Autodesk Inventor part; units mm, degrees
ref_plane "YZ Plane" through (0, 0, 0) normal (1, 0, 0) x (0, 1, 0)
ref_plane "XZ Plane" through (0, 0, 0) normal (0, 1, 0) x (-1, 0, 0)
ref_plane "XY Plane" through (0, 0, 0) normal (0, 0, 1) x (1, 0, 0)
sketch "スケッチ1" plane through (0, 0, 0) normal (0, 0, 1) x (1, 0, 0)
  circle A0 centre (55.7151, -22.426) radius 1
  circle A1 centre (55.7151, -6.426) radius 1.05
  circle A2 centre (20.7151, -6.426) radius 1
  circle A3 centre (4.7151, -6.426) radius 1.45
  circle A4 centre (-30.2849, -22.426) radius 1
  circle A5 centre (-30.2849, -6.426) radius 1.05
  circle A6 centre (55.7151, -22.426) radius 1.1
  circle A7 centre (55.7151, -6.426) radius 1.1
  circle A8 centre (20.7151, -6.426) radius 1.1
  circle A9 centre (4.7151, -6.426) radius 1.1
  circle A10 centre (-30.2849, -6.426) radius 1.1
  circle A11 centre (-30.2849, -22.426) radius 1.1
  circle A12 centre (20.7151, -42.426) radius 1
  circle A13 centre (4.7151, -42.426) radius 1
  circle A14 centre (20.7151, -42.426) radius 1.1
  circle A15 centre (4.7151, -42.426) radius 1.1
  circle A16 centre (55.7151, -6.426) radius 2.5
  circle A17 centre (-30.2849, -6.426) radius 2.5
  circle A18 centre (-30.2849, -22.426) radius 2.5
  circle A19 centre (55.7151, -22.426) radius 2.5
  circle A20 centre (20.7151, -42.426) radius 2.5
  circle A21 centre (4.7151, -42.426) radius 2.5
  line L0 (21.9554, -44.5966) -> (56.9554, -24.5966)
  line L1 (58.2151, -22.426) -> (58.2151, -6.426)
  line L2 (55.7151, -3.926) -> (-30.2849, -3.926)
  line L3 (-32.7849, -6.426) -> (-32.7849, -22.426)
  line L4 (3.4747, -44.5966) -> (-31.5253, -24.5966)
  line L5 (20.7151, -44.926) -> (4.7151, -44.926)
  circle A22 centre (91.7151, -22.426) radius 1
  circle A23 centre (91.7151, -22.426) radius 1.1
  circle A24 centre (-66.2849, -22.426) radius 1.05
  circle A25 centre (-66.2849, -22.426) radius 1.1
  circle A26 centre (-66.2849, -22.426) radius 2.5
  circle A27 centre (91.7151, -22.426) radius 2.5
  line L6 (92.3929, -24.8324) -> (21.3929, -44.8324)
  line L7 (91.7151, -19.926) -> (55.7151, -19.926)
  line L8 (73.8937, -20.8546) -> (67.5365, -20.8546)
  line L9 (73.8937, -16.9974) -> (73.8937, -20.8546)
  line L10 (67.5365, -16.9974) -> (73.8937, -16.9974)
  line L11 (67.5365, -20.8546) -> (67.5365, -16.9974)
  line L12 (73.8937, -20.8546) -> (67.5365, -20.8546)
  line L13 (67.6151, -17.226) -> (73.6151, -17.226)
  line L14 (73.6151, -17.226) -> (73.6151, -20.726)
  line L15 (73.6151, -20.726) -> (67.6151, -20.726)
  line L16 (67.6151, -20.726) -> (67.6151, -17.226)
  line L17 (65.6151, -22.726) -> (75.6151, -22.726)
  line L18 (75.6151, -22.726) -> (75.6151, -15.226)
  line L19 (75.6151, -15.226) -> (65.6151, -15.226)
  line L20 (65.6151, -15.226) -> (65.6151, -22.726)
  line L21 (-66.9603, -24.833) -> (3.4747, -44.5966)
  line L22 (-30.2849, -19.926) -> (-66.2849, -19.926)
  line L23 (-48.4635, -20.8546) -> (-48.4635, -16.9974)
  line L24 (-28.7849, -24.426) -> (-67.7849, -24.426)
  arc A28 (-28.7849, -24.426) -> (-28.2849, -23.926) centre (-28.7849, -23.926) ccw
  line L25 (-28.2849, -4.926) -> (-28.2849, -23.926)
  arc A29 (-28.2849, -4.926) -> (-28.7849, -4.426) centre (-28.7849, -4.926) ccw
  line L26 (-67.7849, -4.426) -> (-28.7849, -4.426)
  arc A30 (-67.7849, -4.426) -> (-68.2849, -4.926) centre (-67.7849, -4.926) ccw
  line L27 (-68.2849, -23.926) -> (-68.2849, -4.926)
  arc A31 (-68.2849, -23.926) -> (-67.7849, -24.426) centre (-67.7849, -23.926) ccw
  line L28 (-48.4635, -7.9974) -> (-42.1063, -7.9974)
  line L29 (-42.1063, -7.9974) -> (-42.1063, -11.8546)
  line L30 (-42.1063, -11.8546) -> (-48.4635, -11.8546)
  line L31 (-48.4635, -11.8546) -> (-48.4635, -7.9974)
  circle A32 centre (-40.8849, -14.426) radius 1.1519
  line L32 (-48.4635, -20.8546) -> (-48.4635, -16.9974)
  line L33 (-48.4635, -16.9974) -> (-42.1063, -16.9974)
  line L34 (-42.1063, -16.9974) -> (-42.1063, -20.8546)
  line L35 (-42.1063, -20.8546) -> (-48.4635, -20.8546)
  circle A33 centre (-66.2849, -6.426) radius 1.8131
  circle A34 centre (-66.2849, -22.426) radius 1.8131
  circle A35 centre (-30.2849, -6.426) radius 1.8131
  circle A36 centre (-30.2849, -22.426) radius 1.8131
  arc A37 (-59.7956, -8.176) -> (-59.7849, -20.676) centre (-59.7849, -14.426) ccw
  arc A38 (-60.0349, -7.926) -> (-59.7956, -8.1758) centre (-59.7849, -7.926) ccw
  line L36 (-60.0349, -7.926) -> (-60.0349, -6.176)
  arc A39 (-59.5349, -6.176) -> (-60.0349, -6.176) centre (-59.7849, -6.176) ccw
  line L37 (-59.5349, -6.176) -> (-59.5349, -7.926)
  arc A40 (-59.7849, -8.176) -> (-59.5349, -7.926) centre (-59.7849, -7.926) ccw
  arc A41 (-57.3931, -8.6518) -> (-59.7849, -8.176) centre (-59.7849, -14.426) ccw
  arc A42 (-57.5284, -8.3251) -> (-57.3931, -8.6518) centre (-57.2975, -8.4208) ccw
  line L38 (-57.5284, -8.3251) -> (-56.8587, -6.7083)
  arc A43 (-56.3968, -6.8997) -> (-56.8587, -6.7083) centre (-56.6278, -6.804) ccw
  line L39 (-56.3968, -6.8997) -> (-57.0665, -8.5165)
  arc A44 (-57.3931, -8.6518) -> (-57.0665, -8.5165) centre (-57.2975, -8.4208) ccw
  arc A45 (-55.3655, -10.0066) -> (-57.3931, -8.6518) centre (-59.7849, -14.426) ccw
  arc A46 (-55.3655, -9.653) -> (-55.3655, -10.0066) centre (-55.1887, -9.8298) ccw
  line L40 (-55.3655, -9.653) -> (-54.1281, -8.4156)
  arc A47 (-53.7745, -8.7692) -> (-54.1281, -8.4156) centre (-53.9513, -8.5924) ccw
  line L41 (-53.7745, -8.7692) -> (-55.0119, -10.0066)
  arc A48 (-55.3655, -10.0066) -> (-55.0119, -10.0066) centre (-55.1887, -9.8298) ccw
  arc A49 (-54.0107, -12.0342) -> (-55.3655, -10.0066) centre (-59.7849, -14.426) ccw
  arc A50 (-53.8754, -11.7076) -> (-54.0107, -12.0342) centre (-53.7797, -11.9386) ccw
  line L42 (-53.8754, -11.7076) -> (-52.2586, -11.0379)
  arc A51 (-52.0672, -11.4998) -> (-52.2586, -11.0379) centre (-52.1629, -11.2689) ccw
  line L43 (-52.0672, -11.4998) -> (-53.684, -12.1695)
  arc A52 (-54.0107, -12.0342) -> (-53.684, -12.1695) centre (-53.7797, -11.9386) ccw
  arc A53 (-53.5349, -14.426) -> (-54.0107, -12.0342) centre (-59.7849, -14.426) ccw
  arc A54 (-53.2849, -14.176) -> (-53.5349, -14.426) centre (-53.2849, -14.426) ccw
  line L44 (-53.2849, -14.176) -> (-51.5349, -14.176)
  arc A55 (-51.5349, -14.676) -> (-51.5349, -14.176) centre (-51.5349, -14.426) ccw
  line L45 (-51.5349, -14.676) -> (-53.2849, -14.676)
  arc A56 (-53.5349, -14.426) -> (-53.2849, -14.676) centre (-53.2849, -14.426) ccw
  arc A57 (-54.0107, -16.8178) -> (-53.5349, -14.426) centre (-59.7849, -14.426) ccw
  arc A58 (-53.684, -16.6825) -> (-54.0107, -16.8178) centre (-53.7797, -16.9134) ccw
  line L46 (-53.684, -16.6825) -> (-52.0672, -17.3522)
  arc A59 (-52.2586, -17.8141) -> (-52.0672, -17.3522) centre (-52.1629, -17.5831) ccw
  line L47 (-52.2586, -17.8141) -> (-53.8754, -17.1444)
  arc A60 (-54.0107, -16.8178) -> (-53.8754, -17.1444) centre (-53.7797, -16.9134) ccw
  arc A61 (-55.3655, -18.8454) -> (-54.0107, -16.8178) centre (-59.7849, -14.426) ccw
  arc A62 (-55.0119, -18.8454) -> (-55.3655, -18.8454) centre (-55.1887, -19.0222) ccw
  line L48 (-55.0119, -18.8454) -> (-53.7745, -20.0829)
  arc A63 (-54.1281, -20.4364) -> (-53.7745, -20.0829) centre (-53.9513, -20.2596) ccw
  line L49 (-54.1281, -20.4364) -> (-55.3655, -19.199)
  arc A64 (-55.3655, -18.8454) -> (-55.3655, -19.199) centre (-55.1887, -19.0222) ccw
  arc A65 (-57.3931, -20.2003) -> (-55.3655, -18.8454) centre (-59.7849, -14.426) ccw
  arc A66 (-57.0665, -20.3356) -> (-57.3931, -20.2003) centre (-57.2975, -20.4312) ccw
  line L50 (-57.0665, -20.3356) -> (-56.3968, -21.9523)
  arc A67 (-56.8587, -22.1437) -> (-56.3968, -21.9523) centre (-56.6278, -22.048) ccw
  line L51 (-56.8587, -22.1437) -> (-57.5284, -20.5269)
  arc A68 (-57.3931, -20.2003) -> (-57.5284, -20.5269) centre (-57.2975, -20.4312) ccw
  arc A69 (-59.7849, -20.676) -> (-57.3931, -20.2003) centre (-59.7849, -14.426) ccw
  arc A70 (-59.5349, -20.926) -> (-59.7849, -20.676) centre (-59.7849, -20.926) ccw
  line L52 (-59.5349, -20.926) -> (-59.5349, -22.676)
  arc A71 (-60.0349, -22.676) -> (-59.5349, -22.676) centre (-59.7849, -22.676) ccw
  line L53 (-60.0349, -22.676) -> (-60.0349, -20.926)
  arc A72 (-59.7849, -20.676) -> (-60.0349, -20.926) centre (-59.7849, -20.926) ccw
  line L54 (-50.4635, -22.8546) -> (-40.1063, -22.8546)
  line L55 (-40.1063, -22.8546) -> (-40.1063, -14.9974)
  line L56 (-40.1063, -14.9974) -> (-50.4635, -14.9974)
  line L57 (-50.4635, -22.8546) -> (-50.4635, -14.9974)
  circle A73 centre (-59.7849, -14.426) radius 8
  circle A74 centre (85.2151, -14.426) radius 8
  point P0 (0, 0)
  point P1 (-32.7849, -19.926)
  point P2 (-40.1063, -19.926)
  point P3 (-50.4635, -19.926)
  point P4 (-53.9314, -19.926)
  point P5 (-54.3076, -20.2569)
  point P6 (-56.494, -21.7178)
  point P7 (-56.9559, -21.9091)
  point P8 (-59.5349, -22.4221)
  point P9 (-60.0349, -22.4221)
  point P10 (-65.4578, -20.0668)
  point P11 (65.6151, -19.926)
  point P12 (58.2151, -19.926)
  point P13 (90.888, -20.0668)
  point P14 (79.4056, -19.926)
  point P15 (75.6151, -19.926)
  dimension "d0" = 2.2
  dimension "d1" = 2.2
  dimension "d2" = 2.2
  dimension "d3" = 2.2
  dimension "d4" = 2.2
  dimension "d5" = 2.2
  dimension "d6" = 2.2
  dimension "d7" = 2.2
  dimension "d8" = 5
  dimension "d9" = 5
  dimension "d10" = 5
  dimension "d11" = 5
  dimension "d12" = 5
  dimension "d13" = 5
  dimension "d18" = 2.2
  dimension "d19" = 2.2
  dimension "d20" = 5
  dimension "d21" = 5
  dimension "d22" = 2
  dimension "d23" = 2
  dimension "d24" = 2
extrude "押し出し1" add sketch "スケッチ1" along normal blind 1.5 contours A3 | A16 | L1 L7 A19 L0 A20 L5 A21 L4 A18 A28 L25 A17 A29 L2 A16 | L7 L20 L17 L18 A74 A27 L6 A20 L0 A19 L1 | L1 A19 L7 | A17 L26 | A19 | A29 A17 | A17 L25 L26 | A17 L25 | A17 L25 A18 L22 L3 | A20 | L22 A18 L3 | L3 A18 L24 A26 A73 L53 A71 L52 L51 A67 L50 L49 A63 L48 L22 L57 L54 L55 | L25 A18 L24 | A18 L25 | L27 A26 | A26 A73 L24 L27 | A27 A74 | A28 A18 | L24 A18 | A18 L4 L21 A26 L24 | A21 | A26 L24 | A34 | A35 | A36 picked at (89.8821, -21.5749)
sketch "スケッチ2" plane through (0, 0, 1.5) normal (0, 0, 1) x (1, 0, 0)
  circle A0 centre (12.7151, -12.926) radius 8
  point P0 (0, 0)
extrude "押し出し2" cut sketch "スケッチ2" against normal through all
fillet "フィレット1" radius 2 8 edges at (75.6151, -19.926, 0.75) (75.6151, -22.726, 0.75) (65.6151, -22.726, 0.75) (65.6151, -19.926, 0.75) (-50.4635, -19.926, 0.75) (-50.4635, -22.8546, 0.75) (-40.1063, -22.8546, 0.75) (-40.1063, -19.926, 0.75)
properties part number "jouhansin_sita"
Geometry: final body of the model. Coordinates: model frame, mm. Coordinates: 2 decimals unless noted, no trailing zeros. Order: outer loops, then holes, each group sorted by start corner. A loop starts at its lowest first (then second) coordinate and runs counter-clockwise, first axis right, second up.
(1) First-contact query: pin 1 (2.5 mm diameter, centred on x = -30.28, y = -22.43, fed in from +Z); pin 2 (2 mm diameter, centred on x = 4.72, y = -42.43, fed in from +Z); pin 3 (0.8 mm diameter, centred on y = -11.5, z = 0.5, fed in from +X). Flat tips, straight axial feed; report the tip coordinate or a pass-through.
(2) Section query A-A (x = 17). Return the cut outline in (y, z).
(3) Draft query along Y for faces 1 (the face through (57.39, -34.692, 0.74)), 2 (the face through (12, -24, 0)), 3 (the face through (17.016, -6.18, 0.76)), 4 (the face through (-68.685, -21.728, 0.74)). Return one class per face: pulls with the +Y half, pulls with the -Y half, needs draft (parallel to the pull), parting line crosses it, or undercut.
(4) Section query B-B (y = -18). Return the cut outline in (x, z), plus the area to 3 significant figures.
(5) Section query C-C (z = 0.65). State how many separate pieces and enclosed holes the cut face has, plus the area to 3 significant figures.
(6) Material intervals for probe 1 along Y at (x, z) = (-30, 1.1); probe 2 along Y at (x, z) = (5.5, 0.5); probe 3 along Y at (x, z) = (56, 0.5), sorted ascending.
(7) Section query D-D (x = -11). Return the cut outline in (y, z), plus the area to 3 significant figures.
Solution:
1. pin 1: stops at z = 1.5
1. pin 2: passes through
1. pin 3: stops at x = 58.22
2. outline: (-44.93, 0) - (-19.68, 0) - (-19.68, 1.5) - (-44.93, 1.5) - close; (-6.17, 0) - (-3.93, 0) - (-3.93, 1.5) - (-6.17, 1.5) - close
3. face 1: pulls with the -Y half
3. face 2: needs draft
3. face 3: undercut
3. face 4: parting line crosses it
4. outline: (-32.78, 0) - (6.53, 0) - (6.53, 1.5) - (-32.78, 1.5) - close; (18.9, 0) - (58.22, 0) - (58.22, 1.5) - (18.9, 1.5) - close
4. area: 118 mm2
5. separate pieces: 1
5. enclosed holes: 11
5. area: 3,680 mm2
6. probe 1: y = -35.2 to -23.49, -21.36 to -7.49, -5.36 to -3.93
6. probe 2: y = -44.93 to -43.2, -41.66 to -16.38, -9.47 to -7.2, -5.66 to -3.93
6. probe 3: y = -35.08 to -23.49, -21.36 to -7.49, -5.36 to -3.94
7. outline: (-40.54, 0) - (-3.93, 0) - (-3.93, 1.5) - (-40.54, 1.5) - close
7. area: 54.9 mm2
